Autodesk Inventor part; units mm, degrees
ref_plane "YZ Plane" through (0, 0, 0) normal (1, 0, 0) x (0, 1, 0)
ref_plane "XZ Plane" through (0, 0, 0) normal (0, 1, 0) x (-1, 0, 0)
ref_plane "XY Plane" through (0, 0, 0) normal (0, 0, 1) x (1, 0, 0)
sketch "Sketch1" plane through (0, 0, 0) normal (0, 1, 0) x (-1, 0, 0)
  line L0 (0, 0) -> (0, 97.9)
  line L1 (68.1, 97.9) -> (91.9, 97.9)
  line L2 (0, 97.9) -> (68.1, 97.9) construction
  line L3 (91.9, 97.9) -> (91.9, 0)
  line L4 (91.9, 0) -> (80, 0)
  line L5 (80, 0) -> (80, 86)
  line L6 (80, 0) -> (0, 0) construction
  line L7 (-406, 406) -> (-308.1, 406)
  line L8 (-308.1, 406) -> (-308.1, 337.9) construction
  line L9 (-406, 314.1) -> (-406, 326)
  line L10 (-406, 326) -> (-320, 326)
  line L11 (-406, 326) -> (-406, 406) construction
  line L12 (-308.1, 406) -> (0, 406) construction
  line L13 (0, 406) -> (0, 97.9) construction
  line L14 (68.1, 97.9) -> (68.1, 86)
  line L15 (68.1, 86) -> (80, 86)
  line L16 (-308.1, 337.9) -> (-320, 337.9)
  line L17 (-320, 337.9) -> (-320, 326)
  line L18 (-406, 314.1) -> (-308.1, 314.1)
  line L19 (-308.1, 337.9) -> (-308.1, 314.1)
  line L20 (-320, 337.9) -> (-320, 406) construction
  line L21 (68.1, 86) -> (0, 86) construction
  dimension "d0" = 160
  dimension "d1" = 11.9
  dimension "d2" = 86
  dimension "d4" = 136.2
  dimension "d6" = 160
  dimension "d7" = 136.2
  dimension "d10" = 11.9
  dimension "d11" = 11.9
  dimension "d12" = 86
  dimension "d14" = 320
  dimension "d15" = 320
  dimension "d16" = 11.9
revolve "Revolution1" add sketch "Sketch1" angle 360 about axis through (0, 0, 0) along (0, 0, 1) contours L1 L3 L4 L5 L15 L14
sketch "Sketch2" plane through (0, 0, 0) normal (0, 1, 0) x (-1, 0, 0)
  line L0 (0, 97.9) -> (0, 406) construction
  line L1 (0, 406) -> (-308.1, 406) construction
  arc A0 (0, 97.9) -> (-308.1, 406) centre (-308.1, 97.9) ccw
  line L2 (-91.9, 97.9) -> (91.9, 97.9)
  dimension "d8" = 308.1
  dimension "d9" = 308.1
sketch "Sketch3" plane through (0, 0, 97.9) normal (0, 0, 1) x (1, 0, 0)
  circle A0 centre (0, 0) radius 80
  circle A1 centre (0, 0) radius 80
  circle A2 centre (0, 0) radius 68.1
  circle A3 centre (0, 0) radius 68.1
  dimension "d13" = 160
sweep "Sweep1" add profiles "Sketch3" path "Sketch2" path curves A0
revolve "Revolution2" add sketch "Sketch1" angle 360 about axis through (406, 0, 406) along (-1, 0, 0) contours L9 L10 L17 L16 L19 L18
equation "\"d0\" = D1"
equation "\"d1\" = S"
equation "\"d2\" = T"
equation "\"d4\" = D1 - 2 * S"
equation "\"d6\" = D1"
equation "\"d7\" = D1 - 2 * S"
equation "\"d10\" = S"
equation "\"d11\" = S"
equation "\"d12\" = T"
equation "\"d14\" = Z"
equation "\"d15\" = Z"
equation "\"d16\" = S"
equation "\"d8\" = Z - S"
equation "\"d9\" = Z - S"
equation "\"d13\" = D1"
equation "\"D1\" = 160"
equation "\"T\" = 86"
equation "\"Z\" = 320"
equation "\"S\" = 11.9"
properties part number "DIN 8063 Колено 90 градусов, тип B 160" material "ПВХ, непластифицированный"
The listing builds one solid part. Answer for the finished solid, in the listing's coordinates (mm). A direction names the side the tool comes from. Round coordinates to 2 decimals unless told otherwise and drop trailing zeros. Loops run counter-clockwise (first coordinate to the right, second up) from the corner with the lowest first, then second, coordinate; pieces in that order, holes last. Notation, with made-up numbers: (50.25, 82) - (83.25, 82) arc R30 ccw to (83.25, 116) - close; hole circle Ø7 at (73.5, 50). An arc over 180 degrees is marked (long way). Use one line per item in the form item = value. Start each with the question number.
1. Consider line 1 (Y direction, x = 314, z = 406); line 2 (Z direction, x = 357.5, y = 0); line 3 (Y direction, x = 371, z = 406). Determine where each line is inside the solid, lowest interval first. Write a range as [from, to].
2. For a pull along Y with two mould halves and no side action, classify faces 1 (the face through (356.36, -4.04, 497.81)), 2 (the face through (54.04, -41.44, 91.87)), 3 (the face through (406, -75.3, 433.7)) as pulls with the +Y half, pulls with the -Y half, needs draft (parallel to the pull), parting line crosses it, or undercut.
3. The part is cut by section B-B on x = 338.5. Determine the outline of the cut face in (y, z), then the cut area to 3 significant figures.
4. The part is cut by section A-A on y = 0. Determine the outline of the cut face in (x, z), then the cut area to 3 significant figures.
5. A tool of negligible diameter and unlimited length cuts with its end or side. For faces 4 (the face through (314.1, -26.1, 343.1)), 5 (the face through (308.1, -75.3, 433.7)), 6 (the face through (-59, -36, 86)), from which of +Z, -Z, +X, -X, +Y, -Y can it reach the whole face along a straight path? Write none if from no direction.
6. The part is cut by section C-C on z = 76. Determine the outline of the cut face in (x, y), then the cut area to 3 significant figures.
7. The part is cut by section D-D on y = 32.5. Determine the outline of the cut face in (x, z).
8. Given pin 1 Ø2 at (y, z) = (-21, 448) entering from -X; pin 2 Ø2 at (y, z) = (2, 374.5) entering from +X; pin 3 Ø12 at (x, y) = (172.5, -49) entering from -Z, each flat-ended and moving along its own axis, determine where each tip first touches the part or whether it passes through.
Geometry check:
q1.line_1 = [-91.9, -68.1], [68.1, 91.9]
q1.line_2 = [314.1, 326], [486, 497.9]
q1.line_3 = [-91.9, -80], [80, 91.9]
q2.face_1 = parting line crosses it
q2.face_2 = undercut
q2.face_3 = needs draft
q3.outline = circle Ø183.8 at (0, 406); hole circle Ø160 at (0, 406)
q3.area = 6,430 mm^2
q4.outline = (-91.9, 0) - (-80, 0) - (-80, 86) - (-68.1, 86) - (-68.1, 97.9) arc R376.2 cw to (308.1, 474.1) - (320, 474.1) - (320, 486) - (406, 486) - (406, 497.9) - (308.1, 497.9) - (308.1, 486) arc R388.1 ccw to (-80, 97.9) - (-91.9, 97.9) - close; (68.1, 86) - (80, 86) - (80, 0) - (91.9, 0) - (91.9, 97.9) - (80, 97.9) arc R228.1 cw to (308.1, 326) - (308.1, 314.1) - (406, 314.1) - (406, 326) - (320, 326) - (320, 337.9) - (308.1, 337.9) arc R240 ccw to (68.1, 97.9) - close
q4.area = 16,700 mm^2
q5.face_4 = +X
q5.face_5 = none
q5.face_6 = -Z
q6.outline = circle Ø183.8 at (0, 0); hole circle Ø160 at (0, 0)
q6.area = 6,430 mm^2
q7.outline = (-85.96, 0) - (-73.1, 0) - (-73.1, 86) - (-59.84, 86) - (-59.84, 97.9) arc R367.94 cw to (308.1, 465.84) - (320, 465.84) - (320, 479.1) - (406, 479.1) - (406, 491.96) - (308.1, 491.96) - (308.1, 479.1) arc R381.2 ccw to (-73.1, 97.9) - (-85.96, 97.9) - close; (59.84, 86) - (73.1, 86) - (73.1, 0) - (85.96, 0) - (85.96, 97.9) - (73.1, 97.9) arc R235 cw to (308.1, 332.9) - (308.1, 320.04) - (406, 320.04) - (406, 332.9) - (320, 332.9) - (320, 346.16) - (308.1, 346.16) arc R248.26 ccw to (59.84, 97.9) - close
q8.pin_1 = 144.97
q8.pin_2 = 54.25
q8.pin_3 = 295.13
